```python
from build123d import *

# Parameters (mm, degrees)
FILLET1_R               = 3
SKETCH2_W               = 23.002294749
SKETCH2_H               = 32.038910542
CUT_EXTRUDE1_DEPTH      = 30
SKETCH3_R               = 6.178270045
CUT_EXTRUDE2_DEPTH      = 20
SKETCH4_R               = 10
CUT_EXTRUDE3_DEPTH      = 30
CUT_EXTRUDE4_DEPTH      = 137.747943453
CUT_EXTRUDE4_DEPTH_BACK = 33


with BuildPart() as part:
    # Sketch1 → Revolve1 (revolve)
    with BuildSketch(Plane.XY, mode=Mode.PRIVATE) as revolve1_sk:
        Polygon((0, 0), (-60, 0), (-60, 15), (0, 15), (0, 30), (50, 30), (50, 25), (130, 25), (130, 0), align=None)
    revolve(revolve1_sk.sketch.rotate(Axis((-83.2159872, 0, 0), (1, 0, 0)), 180), axis=Axis((-83.2159872, 0, 0), (1, 0, 0)))

    # Fillet1
    fillet1_edges = [part.edges().sort_by_distance(p)[0] for p in [
        (130, 25, 0),
    ]]
    fillet(fillet1_edges, radius=FILLET1_R)

    # Sketch2 → Cut-Extrude1 (cut)
    with BuildSketch(Plane.XY):
        with Locations((79.66963489, 1.540332238)):
            Rectangle(SKETCH2_W, SKETCH2_H)
    extrude(amount=-CUT_EXTRUDE1_DEPTH, mode=Mode.SUBTRACT)

    # Sketch3 → Cut-Extrude2 (cut)
    with BuildSketch(Plane(origin=(0, 0, 0), x_dir=(-1, 0, 0), z_dir=(0, 0, -1))):
        with Locations((-79.938300401, 1.139218287)):
            Circle(SKETCH3_R)
    extrude(amount=-CUT_EXTRUDE2_DEPTH, mode=Mode.SUBTRACT)

    # Sketch4 → Cut-Extrude3 (cut)
    with BuildSketch(Plane.XY):
        with Locations((24.012296705, 2.977975659)):
            Circle(SKETCH4_R)
    extrude(amount=-CUT_EXTRUDE3_DEPTH, mode=Mode.SUBTRACT)

    # Sketch6 → Cut-Extrude4 (cut, two sides: drawn at the far end of the back side and taken through both)
    with BuildSketch(Plane.XY.offset(-CUT_EXTRUDE4_DEPTH_BACK)):
        with BuildLine():
            Line((-35, 4.826374344), (-20, 4.826374344))
            ThreePointArc((-20, 4.826374344), (-15.173625656, 0), (-20, -4.826374344))
            Line((-20, -4.826374344), (-35, -4.826374344))
            ThreePointArc((-35, -4.826374344), (-39.826374344, 0), (-35, 4.826374344))
        make_face()
    extrude(amount=CUT_EXTRUDE4_DEPTH + CUT_EXTRUDE4_DEPTH_BACK, mode=Mode.SUBTRACT)


solid = part.part
```
Model file for the job. Use its own axes, mm. A direction names the side the tool comes from. Coordinates: 2 decimals unless noted, no trailing zeros. Write each loop counter-clockwise with the first axis right and the second up, starting at its lowest first coordinate (ties: lowest second). Pieces come first, ordered by that corner, then holes. Notation, with made-up numbers: (-17, 34.5) - (8, 34.5) arc R15 ccw to (8, 44.5) - close; hole circle Ø3 at (38, -30.75). An arc over 180 degrees is marked (long way). One line per item, written item: value. Start each with the question number.
1. Tool access for faces 5 (the flat face through (80, 17.56, -9)), 6 (the flat face through (-27, -4.826, 0)), 7 (the flat face through (50, 7, -25)): list every direction of +Z, -Z, +X, -X, +Y, -Y with a clear straight run to the whole face (end or side of a thin tool).
2. Slice it at A-A (x = -26). Write the cut outline in (y, z).
3. Flat gauge pins, fed straight in: pin 1 (3 mm diameter, centred on x = 33, z = 21.5, fed in from +Y); pin 2 (8 mm diameter, centred on x = 34, z = 20, fed in from -Y); pin 3 (3 mm diameter, centred on x = 109, y = 21, fed in from -Z). Where does each tip first touch, or does it go through?
4. Mould opens along Y. For faces 1 (the flat face through (74, 5, 0)), 2 (the flat face through (0, 6, -14)), 3 (the cylindrical face through (25.35, -13.843, 26.615)), 4 (the cylindrical face through (-39.825, -0.106, -0.21)) say: released by +Y, released by -Y, zero draft, split by the parting line, or undercut.
5. Slice it at C-C (x = 117). Write the cut outline in (y, z).
6. Slice it at B-B (z = 4). Count the separate pieces of the cut face and the enclosed holes in it, plus the area to 3 significant figures.
7. Probe line 1 (X direction, y = 5.5, z = -15); line 2 (X direction, y = 10, z = -18.5); line 3 (X direction, y = -13, z = 15.5). List the from-to ranges inside material, lowest first. Write a range as from..to.
Answers below:
1. face 5: -Z
1. face 6: +Z, -Z
1. face 7: +X
2. outline: (-4.83, -14.2) - (-4.83, 14.2) arc R15 ccw to start; (4.83, -14.2) arc R15 ccw to (4.83, 14.2) - close
3. pin 1: stops at y = 22.36
3. pin 2: stops at y = -25.38
3. pin 3: stops at z = -15.64
4. face 1: undercut
4. face 2: zero draft
4. face 3: split by the parting line
4. face 4: undercut
5. outline: circle Ø50 at (0, 0)
6. separate pieces: 1
6. enclosed holes: 2
6. area: 8,310 mm^2
7. line 1: x = 0..14.34, 33.69..68.17, 91.17..130
7. line 2: x = 0..16.89, 31.13..68.17, 91.17..130
7. line 3: x = 0..130
